Can you work these out from the model? Positions are in its coordinate system, mm. A direction names the side the tool comes from. Coordinates: 2 decimals unless noted, no trailing zeros. Write each loop counter-clockwise with the first axis right and the second up, starting at its lowest first coordinate (ties: lowest second). Pieces come first, ordered by that corner, then holes. Notation, with made-up numbers: M 70.25,28 L 122.25,28 A22 ccw 122.25,40 Z; hole C 49.5,77 d7. An arc over 180 degrees is marked long. Use one line per item in the form item = value. Start each with the question number.
```python
from build123d import *

# Parameters (mm, degrees)
SKETCH1_R           = 3.4
BOSS_EXTRUDE1_DEPTH = 1
SKETCH2_R           = 2.9
BOSS_EXTRUDE2_DEPTH = 1
CUT_EXTRUDE1_DEPTH  = 6.667450926
FILLET1_R           = 0.4
FILLET2_R           = 0.4
FILLET3_R           = 0.4
FILLET4_R           = 0.4
FILLET5_R           = 0.1
FILLET6_R           = 0.1
FILLET7_R           = 0.1
FILLET8_R           = 0.1
FILLET9_R           = 0.1
FILLET10_R          = 0.1
FILLET11_R          = 0.1
FILLET12_R          = 0.1


with BuildPart() as part:
    # Sketch1 → Boss-Extrude1 (new body)
    with BuildSketch(Plane.XY):
        Circle(SKETCH1_R)
    boss_extrude1 = extrude(amount=BOSS_EXTRUDE1_DEPTH)

    # Sketch2 → Boss-Extrude2 (add)
    with BuildSketch(Plane.XY.offset(1)):
        Circle(SKETCH2_R)
    extrude(amount=BOSS_EXTRUDE2_DEPTH)

    # Mirror3: Boss-Extrude1 across plane
    add(boss_extrude1.mirror(Plane.XY.offset(1.5)))

    # Sketch3 → Cut-Extrude1 (cut, through all)
    with BuildSketch(Plane(origin=(0, 0, 0), x_dir=(-1, 0, 0), z_dir=(0, 0, -1))):
        with BuildLine():
            Line((0.84, -0.84), (0.84, -2.248199279))
            ThreePointArc((0.84, -2.248199279), (0, -2.4), (-0.84, -2.248199279))
            Line((-0.84, -2.248199279), (-0.84, -0.84))
            Line((-0.84, -0.84), (-2.248199279, -0.84))
            ThreePointArc((-2.248199279, -0.84), (-2.4, 0), (-2.248199279, 0.84))
            Line((-2.248199279, 0.84), (-0.84, 0.84))
            Line((-0.84, 0.84), (-0.84, 2.248199279))
            ThreePointArc((-0.84, 2.248199279), (0, 2.4), (0.84, 2.248199279))
            Line((0.84, 2.248199279), (0.84, 0.84))
            Line((0.84, 0.84), (2.248199279, 0.84))
            ThreePointArc((2.248199279, 0.84), (2.4, 0), (2.248199279, -0.84))
            Line((2.248199279, -0.84), (0.84, -0.84))
        make_face()
    extrude(amount=-CUT_EXTRUDE1_DEPTH, mode=Mode.SUBTRACT)

    # Fillet1
    fillet1_edges = [part.edges().sort_by_distance(p)[0] for p in [
        (-0.84, 0.84, 1.5),
    ]]
    fillet(fillet1_edges, radius=FILLET1_R)

    # Fillet2
    fillet2_edges = [part.edges().sort_by_distance(p)[0] for p in [
        (0.84, 0.84, 1.5),
    ]]
    fillet(fillet2_edges, radius=FILLET2_R)

    # Fillet3
    fillet3_edges = [part.edges().sort_by_distance(p)[0] for p in [
        (0.84, -0.84, 1.5),
    ]]
    fillet(fillet3_edges, radius=FILLET3_R)

    # Fillet4
    fillet4_edges = [part.edges().sort_by_distance(p)[0] for p in [
        (-0.84, -0.84, 1.5),
    ]]
    fillet(fillet4_edges, radius=FILLET4_R)

    # Fillet5
    fillet5_edges = [part.edges().sort_by_distance(p)[0] for p in [
        (0.84, -2.248199279, 1.5),
    ]]
    fillet(fillet5_edges, radius=FILLET5_R)

    # Fillet6
    fillet6_edges = [part.edges().sort_by_distance(p)[0] for p in [
        (-0.84, -2.248199279, 1.5),
    ]]
    fillet(fillet6_edges, radius=FILLET6_R)

    # Fillet7
    fillet7_edges = [part.edges().sort_by_distance(p)[0] for p in [
        (-2.248199279, 0.84, 1.5),
    ]]
    fillet(fillet7_edges, radius=FILLET7_R)

    # Fillet8
    fillet8_edges = [part.edges().sort_by_distance(p)[0] for p in [
        (-2.248199279, -0.84, 1.5),
    ]]
    fillet(fillet8_edges, radius=FILLET8_R)

    # Fillet9
    fillet9_edges = [part.edges().sort_by_distance(p)[0] for p in [
        (-0.84, 2.248199279, 1.5),
    ]]
    fillet(fillet9_edges, radius=FILLET9_R)

    # Fillet10
    fillet10_edges = [part.edges().sort_by_distance(p)[0] for p in [
        (0.84, 2.248199279, 1.5),
    ]]
    fillet(fillet10_edges, radius=FILLET10_R)

    # Fillet11
    fillet11_edges = [part.edges().sort_by_distance(p)[0] for p in [
        (2.248199279, 0.84, 1.5),
    ]]
    fillet(fillet11_edges, radius=FILLET11_R)

    # Fillet12
    fillet12_edges = [part.edges().sort_by_distance(p)[0] for p in [
        (2.248199279, -0.84, 1.5),
    ]]
    fillet(fillet12_edges, radius=FILLET12_R)


solid = part.part
```
1) Please list where these lines run through material, in increasing order: line 1 (Z direction, x = 2.5, y = -1.75); line 2 (Y direction, x = 0, z = 0.9); line 3 (Y direction, x = -0.5, z = 1.65).
2) Will these pins go through, and if not, where does the flat tip stop? pin 1 Ø0.8 at (y, z) = (-1.5, 2) entering from -X; pin 2 Ø0.8 at (y, z) = (-1.5, 1) entering from +X; pin 3 Ø1.5 at (x, z) = (-1.5, 0.5) entering from -Y.
3) Suppose I cut it at D-D on z = 1.65. Please give me the cut outline in (x, y).
4) Suppose I cut it at B-B on z = 2.7. Please give me the cut outline in (x, y).
5) If we mould it in two halves opening along Y, with no side actions, what happens to faces 4 (the face through (0.84, 2, 1)), 5 (the face through (-2.9, 0.1, 1.5)), 6 (the face through (3, 1, 1))? For each: +Y half, -Y half, draft (parallel to the pull), parting line (faces both ways), or undercut.
6) Suppose I cut it at A-A on x = 0. Please give me the cut outline in (y, z), and give its area (3 significant figures).
7) Which directions (+Z, -Z, +X, -X, +Y, -Y) give clear straight access to the entire face, cutting with the end or side of a thin tool? Please do faces 1 (the face through (-2, -0.84, 1)), 2 (the face through (1.5, -1.5, 0)), 3 (the face through (3, 1, 2)).
Computed values:
q1.line_1 = 0 to 1, 2 to 3
q1.line_2 = -3.4 to -2.4, 2.4 to 3.4
q1.line_3 = -2.86 to -2.35, 2.35 to 2.86
q2.pin_1 = -3.22
q2.pin_2 = 3.22
q2.pin_3 = -3.32
q3.outline = C 0,0 d5.8; hole M -2.27,-0.77 A0.1 ccw -2.18,-0.84 L -1.24,-0.84 A0.4 cw -0.84,-1.24 L -0.84,-2.18 A0.1 ccw -0.77,-2.27 A2.4 ccw 0.77,-2.27 A0.1 ccw 0.84,-2.18 L 0.84,-1.24 A0.4 cw 1.24,-0.84 L 2.18,-0.84 A0.1 ccw 2.27,-0.77 A2.4 ccw 2.27,0.77 A0.1 ccw 2.18,0.84 L 1.24,0.84 A0.4 cw 0.84,1.24 L 0.84,2.18 A0.1 ccw 0.77,2.27 A2.4 ccw -0.77,2.27 A0.1 ccw -0.84,2.18 L -0.84,1.24 A0.4 cw -1.24,0.84 L -2.18,0.84 A0.1 ccw -2.27,0.77 A2.4 ccw Z
q4.outline = C 0,0 d6.8; hole M -2.27,-0.77 A0.1 ccw -2.18,-0.84 L -1.24,-0.84 A0.4 cw -0.84,-1.24 L -0.84,-2.18 A0.1 ccw -0.77,-2.27 A2.4 ccw 0.77,-2.27 A0.1 ccw 0.84,-2.18 L 0.84,-1.24 A0.4 cw 1.24,-0.84 L 2.18,-0.84 A0.1 ccw 2.27,-0.77 A2.4 ccw 2.27,0.77 A0.1 ccw 2.18,0.84 L 1.24,0.84 A0.4 cw 0.84,1.24 L 0.84,2.18 A0.1 ccw 0.77,2.27 A2.4 ccw -0.77,2.27 A0.1 ccw -0.84,2.18 L -0.84,1.24 A0.4 cw -1.24,0.84 L -2.18,0.84 A0.1 ccw -2.27,0.77 A2.4 ccw Z
q5.face_4 = undercut
q5.face_5 = parting line
q5.face_6 = draft
q6.outline = M -3.4,0 L -2.4,0 L -2.4,3 L -3.4,3 L -3.4,2 L -2.9,2 L -2.9,1 L -3.4,1 Z; M 2.4,0 L 3.4,0 L 3.4,1 L 2.9,1 L 2.9,2 L 3.4,2 L 3.4,3 L 2.4,3 Z
q6.area = 5.00 mm²
q7.face_1 = +Z, -Z
q7.face_2 = -Z, +X, -X, +Y, -Y
q7.face_3 = none
